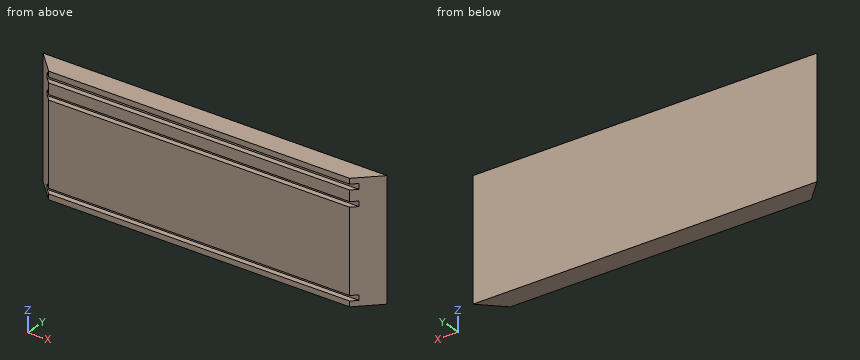
from build123d import *

# Parameters (mm, degrees)
SKETCH2_W           = 203.2
SKETCH2_H           = 12.7
BOSS_EXTRUDE1_DEPTH = 69.85
CHAMFER1_SIZE       = 12.7
SKETCH3_W           = 203.2
SKETCH3_H           = 3.175
SKETCH3_H_2         = 3.000000096
CUT_EXTRUDE2_DEPTH  = 3.175


with BuildPart() as part:
    # Sketch2 → Boss-Extrude1 (new body)
    with BuildSketch(Plane.XY):
        Rectangle(SKETCH2_W, SKETCH2_H)
    extrude(amount=BOSS_EXTRUDE1_DEPTH)

    # Chamfer1
    chamfer1_edges = [part.edges().sort_by_distance(p)[0] for p in [
        (-101.6, -6.35, 34.925),
        (101.6, -6.35, 34.925),
    ]]
    chamfer(chamfer1_edges, length=CHAMFER1_SIZE - 0.0001)  # a hair under: the kernel refuses the full size

    # Sketch3 → Cut-Extrude2 (cut)
    with BuildSketch(Plane.XZ.offset(6.35)):
        with Locations((0, 65.0875)):
            Rectangle(SKETCH3_W, SKETCH3_H)
        with Locations((0, 4.675000048)):
            Rectangle(SKETCH3_W, SKETCH3_H_2)
        with Locations((0, 55.649999952)):
            Rectangle(SKETCH3_W, SKETCH3_H_2)
    extrude(amount=-CUT_EXTRUDE2_DEPTH, mode=Mode.SUBTRACT)


solid = part.part
Could you check a few things on this model? Use its own coordinates, in mm. Give positions to 0.01 mm unless a question says otherwise; leave off trailing zeros. Write each loop counter-clockwise with the first axis right and the second up, starting at its lowest first coordinate (ties: lowest second). Pieces come first, ordered by that corner, then holes. Notation, with made-up numbers: (-30, -14) -> (-12, -14) arc R20 ccw to (-12, -3) -> close; hole circle Ø8 at (30, 30.5). An arc over 180 degrees is marked (long way). Write each question's results on one line, items separated by ' | '. Start each with the question number.
Q1. Suppose I cut it at C-C, the plane y = 0.25. List the corners of the cut face in (x, z) for me, and give its area (3 significant figures).
Q2. I'm going to push flat-ended pins straight in: pin 1 Ø2.5 at (x, z) = (18, 56) entering from -Y; pin 2 Ø5 at (y, z) = (-1.5, 25.5) entering from -X; pin 3 Ø6 at (y, z) = (0.5, 16) entering from -X; pin 4 Ø3 at (y, z) = (-4.5, 9.5) entering from +X. Where does each tip first touch, or does it pass through?
Q3. Suppose I cut it at B-B, the plane x = -4. List the corners of the cut face in (y, z) for me (3 decimals).
Q4. I need wall thicknesses on probe 1 along Z at (x, y) = (-37.5, -4) (3 decimals); probe 2 along Y at (x, z) = (31, 4.5) (3 decimals); probe 3 along X at (y, z) = (1.5, 53.5). Which ranges of each line are inside material? Lowest first, please.
Outcome:
1) outline: (-95.5, 0) -> (95.5, 0) -> (95.5, 69.85) -> (-95.5, 69.85) -> close | area: 13,300 mm2
2) pin 1: y = -6.35 | pin 2: x = -96.25 | pin 3: x = -98.75 | pin 4: x = 92.25
3) outline: (-6.35, 0) -> (6.35, 0) -> (6.35, 69.85) -> (-6.35, 69.85) -> (-6.35, 66.675) -> (-3.175, 66.675) -> (-3.175, 63.5) -> (-6.35, 63.5) -> (-6.35, 57.15) -> (-3.175, 57.15) -> (-3.175, 54.15) -> (-6.35, 54.15) -> (-6.35, 6.175) -> (-3.175, 6.175) -> (-3.175, 3.175) -> (-6.35, 3.175) -> close
4) probe 1: 0 to 3.175, 6.175 to 54.15, 57.15 to 63.5, 66.675 to 69.85 | probe 2: -3.175 to 6.35 | probe 3: -96.75 to 96.75
